```python
from build123d import *

# Parameters (mm, degrees)
ESQUISSE1_W             = 30
ESQUISSE1_H             = 30
BOSS_EXTRU_1_DEPTH      = 38
ESQUISSE2_W             = 17.8
ESQUISSE2_H             = 4.3
ESQUISSE2_W_2           = 4.4
ESQUISSE2_H_2           = 17.8
ENL_V_MAT_EXTRU_1_DEPTH = 26
ESQUISSE5_W             = 26
ESQUISSE5_H             = 4.3
ENL_V_MAT_EXTRU_4_DEPTH = 31


with BuildPart() as part:
    # Esquisse1 → Boss.-Extru.1 (new body)
    with BuildSketch(Plane(origin=(0, 0, 0), x_dir=(1, 0, 0), z_dir=(0, 1, 0))):
        with Locations((-20.886738322, -1.468531469)):
            Rectangle(ESQUISSE1_W, ESQUISSE1_H)
    extrude(amount=BOSS_EXTRU_1_DEPTH)

    # Esquisse2 → Enlèv. mat.-Extru.1 (cut)
    with BuildSketch(Plane.XZ):
        with Locations((-14.786738322, -7.431468531)):
            Rectangle(ESQUISSE2_W, ESQUISSE2_H)
        with Locations((-29.786738322, 7.568531469)):
            Rectangle(ESQUISSE2_W_2, ESQUISSE2_H_2)
        with Locations((-14.786738322, 7.568531469)):
            Rectangle(ESQUISSE2_W, ESQUISSE2_H_2)
    extrude(amount=-ENL_V_MAT_EXTRU_1_DEPTH, mode=Mode.SUBTRACT)

    # Esquisse5 → Enlèv. mat.-Extru.4 (cut, through all)
    with BuildSketch(Plane.ZY.offset(35.886738322)):
        with Locations((3.468531469, 32)):
            Rectangle(ESQUISSE5_W, ESQUISSE5_H)
    extrude(amount=-ENL_V_MAT_EXTRU_4_DEPTH, mode=Mode.SUBTRACT)


solid = part.part
```
Verification items for the finished model (mm, model axes). A direction names the side the tool comes from. Give positions to 0.01 mm unless a question says otherwise; leave off trailing zeros. Write each loop counter-clockwise with the first axis right and the second up, starting at its lowest first coordinate (ties: lowest second). Pieces come first, ordered by that corner, then holes. Notation, with made-up numbers: (-10.5, -32.5) - (-1.5, -32.5) arc R31 cw to (-1.5, 3.5) - close; hole circle Ø6 at (57, 47). An arc over 180 degrees is marked (long way). Put each result on its own line as item: value.
Q1. Section check A-A on z = -5.75. Record the cut outline in (x, y).
Result:
outline: (-35.89, 0) - (-23.69, 0) - (-23.69, 26) - (-5.89, 26) - (-5.89, 29.85) - (-35.89, 29.85) - close; (-35.89, 34.15) - (-5.89, 34.15) - (-5.89, 38) - (-35.89, 38) - close
Q2. Set-up check for faces 1 (the face through (-21, 34.15, 3)), 2 (the face through (-15, 13, -5.281)), 3 (the face through (-31.987, 13, 7)): record each of +Z, -Z, +X, -X, +Y, -Y from which the full face is reachable in a straight line by a thin tool's end or side.
Result:
face 1: +Z, +X, -X
face 2: +X, -Y
face 3: +Z, -Y
Q3. Scan lines: probe 1 along Y at (x, z) = (-18.25, 5.75); probe 2 along X at (y, z) = (25, 8.25); probe 3 along Y at (x, z) = (-27.25, 1.75). Record each from-to range of solid material in increasing order. Write a range as from..to.
Result:
probe 1: 26..29.85, 34.15..38
probe 2: -35.89..-31.99, -27.59..-23.69
probe 3: 0..29.85, 34.15..38
Q4. Section check C-C on y = 10. Record the cut outline in (x, z), and give its area (3 significant figures).
Result:
outline: (-35.89, -13.53) - (-5.89, -13.53) - (-5.89, -9.58) - (-23.69, -9.58) - (-23.69, -5.28) - (-5.89, -5.28) - (-5.89, -1.33) - (-23.69, -1.33) - (-23.69, 16.47) - (-27.59, 16.47) - (-27.59, -1.33) - (-31.99, -1.33) - (-31.99, 16.47) - (-35.89, 16.47) - close
area: 428 mm2
Q5. Section check B-B on x = -9. Record the cut outline in (y, z).
Result:
outline: (0, -13.53) - (38, -13.53) - (38, 16.47) - (34.15, 16.47) - (34.15, -9.53) - (29.85, -9.53) - (29.85, 16.47) - (26, 16.47) - (26, -1.33) - (0, -1.33) - (0, -5.28) - (26, -5.28) - (26, -9.58) - (0, -9.58) - close
Q6. Section check D-D on z = 3.75. Record the cut outline in (x, y), and give its area (3 significant figures).
Result:
outline: (-35.89, 0) - (-31.99, 0) - (-31.99, 26) - (-27.59, 26) - (-27.59, 0) - (-23.69, 0) - (-23.69, 26) - (-5.89, 26) - (-5.89, 29.85) - (-35.89, 29.85) - close; (-35.89, 34.15) - (-5.89, 34.15) - (-5.89, 38) - (-35.89, 38) - close
area: 434 mm2
Q7. Mould release check, pull along Y, two halves, no side actions. Record for faces 4 (the face through (-24, 0, -2)), 5 (the face through (-27, 18, 16.469)), 6 (the face through (-21, 29.85, 3)), 7 (the face through (-21, 32, -9.531)): released by +Y, released by -Y, zero draft, split by the parting line, or undercut.
Result:
face 4: released by -Y
face 5: zero draft
face 6: undercut
face 7: undercut
Q8. Depth check by flat-ended pin: P1, Ø9, axis at x = -11.5, y = 19, coming from the +Z side; P2, Ø1.3, axis at x = -23, y = 33, coming from the +Z side; P3, Ø8, axis at x = -14.5, z = 1, coming from the -Y side; P4, Ø2, axis at y = 14, z = -7, coming from the +X side. Enter the tip coordinate at first touch or a pass-through.
Result:
P1: z = -1.33
P2: z = -9.53
P3: y = 0
P4: x = -23.69
